Study the drawing (mm; zero at the part's minimum x, y, z) and answer. Round coordinates to 2 decimals unless told otherwise and drop trailing zeros. Write each loop counter-clockwise with the first axis right and the second up, starting at its lowest first coordinate (ties: lowest second). Pieces come first, ordered by that corner, then holes.
(1) A cutting plane is placed at A-A, the plane x = 39. Give the vertices of the cut face in (y, z), and give its area (3 significant figures).
(2) A cutting plane is placed at B-B, the plane y = 4. Give the vertices of the cut face in (x, z), and give its area (4 significant figures).
(3) The mould has two halves that part along Y. Classify the marked faces 1, 2 and 3: +Y half, -Y half, draft (parallel to the pull), parting line (faces both ways), or undercut.
(4) A cutting plane is placed at D-D, the plane x = 21. Give the vertices of the cut face in (y, z).
(5) Find the intervals of material crossed by probe 1 along Y at (x, z) = (21, 2.4); probe 2 along X at (y, z) = (3.25, 0.55); probe 3 along X at (y, z) = (5.75, 1.1), in increasing order.
(6) A cutting plane is placed at C-C, the plane z = 1.8. Give the vertices of the cut face in (x, y), and give its area (3 significant figures).
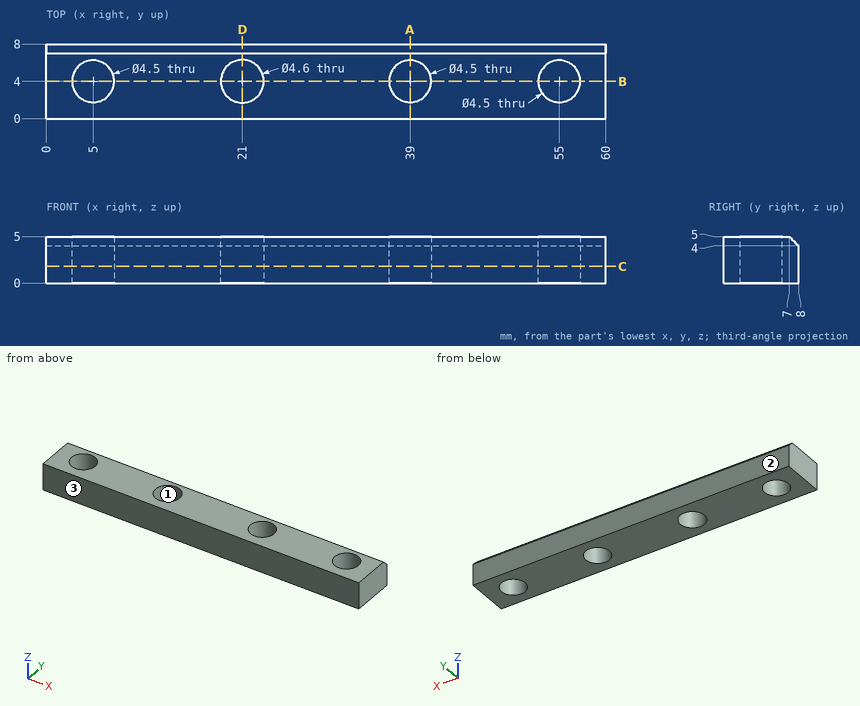
Solutions:
1. outline: (0, 0) - (1.75, 0) - (1.75, 5) - (0, 5) - close; (6.25, 0) - (8, 0) - (8, 4) - (7, 5) - (6.25, 5) - close
1. area: 17.0 mm2
2. outline: (0, 0) - (2.75, 0) - (2.75, 5) - (0, 5) - close; (7.25, 0) - (18.7, 0) - (18.7, 5) - (7.25, 5) - close; (23.3, 0) - (36.75, 0) - (36.75, 5) - (23.3, 5) - close; (41.25, 0) - (52.75, 0) - (52.75, 5) - (41.25, 5) - close; (57.25, 0) - (60, 0) - (60, 5) - (57.25, 5) - close
2. area: 209.5 mm2
3. face 1: undercut
3. face 2: +Y half
3. face 3: -Y half
4. outline: (0, 0) - (1.7, 0) - (1.7, 5) - (0, 5) - close; (6.3, 0) - (8, 0) - (8, 4) - (7, 5) - (6.3, 5) - close
5. probe 1: y = 0 to 1.7, 6.3 to 8
5. probe 2: x = 0 to 2.88, 7.12 to 18.83, 23.17 to 36.88, 41.12 to 52.88, 57.12 to 60
5. probe 3: x = 0 to 3.59, 6.41 to 19.51, 22.49 to 37.59, 40.41 to 53.59, 56.41 to 60
6. outline: (0, 0) - (60, 0) - (60, 8) - (0, 8) - close; hole circle Ø4.5 at (5, 4); hole circle Ø4.6 at (21, 4); hole circle Ø4.5 at (39, 4); hole circle Ø4.5 at (55, 4)
6. area: 416 mm2
